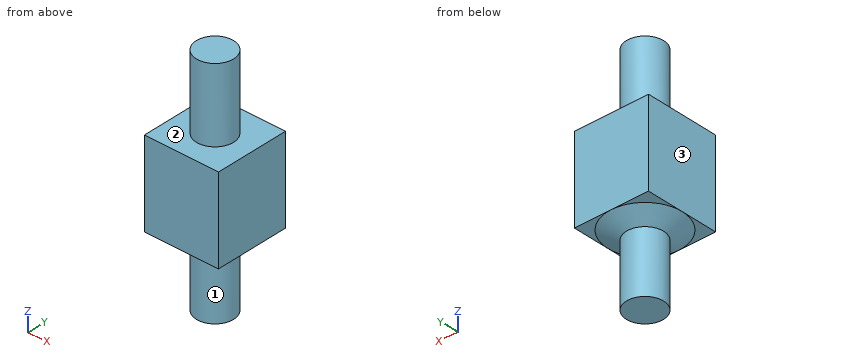
```python
from build123d import *

# Parameters (mm, degrees)
F0_R     = 2
F1_DEPTH = 25
F3_W     = 8
F3_H     = 8
F4_DEPTH = 9.3


with BuildPart() as f1:
    # F0 (on Top) → F1 (new body)
    with BuildSketch(Plane.XY):
        Circle(F0_R)
    extrude(amount=F1_DEPTH)

    # F3 (on offset) → F4 (join)
    with BuildSketch(Plane.XY.offset(17)):
        Rectangle(F3_W, F3_H)
    extrude(amount=-F4_DEPTH)

    # F5 (on Front) → F6 (revolve)
    with BuildSketch(Plane.XZ):
        Polygon((0, 7.7), (0, 5.7), (4, 7.7), align=None)
    revolve(axis=Axis((0, 0, 6.7), (0, 0, -1)))


solid = f1.part
```
Here's how the part is built. I have some questions about the finished solid (model axes, mm). Face numbers are marked on the shaded views. A direction names the side the tool comes from. Round coordinates to 2 decimals unless told otherwise and drop trailing zeros. Order: outer loops, then holes, each group sorted by start corner. A loop starts at its lowest first (then second) coordinate and runs counter-clockwise, first axis right, second up. Notation, with made-up numbers: M -39,-21 L 20,-21 A19 ccw 20,-3 Z; hole C -12,10.5 d8. An arc over 180 degrees is marked long. Answer in a Markdown table with one row per item.
Item 1: For the marked faces 1, 2 and 3, which set-ups out of +Z, -Z, +X, -X, +Y, -Y let a thin tool reach every point of the face, with its end or its side?
A:
| item | result |
|---|---|
| face 1 | -Z |
| face 2 | +Z |
| face 3 | +Z, -Z, -X, +Y, -Y |
Item 2: I'm going to push flat-ended pins straight in: pin 1 (2 mm diameter, centred on x = -2, y = -3, fed in from -Z); pin 2 (1.2 mm diameter, centred on x = -1.5, y = -2.5, fed in from -Z); pin 3 (1 mm diameter, centred on y = 0.5, z = 3.5, fed in from -X). Where does each tip first touch, or does it pass through?
A:
| item | result |
|---|---|
| pin 1 | stops at z = 7 |
| pin 2 | stops at z = 6.86 |
| pin 3 | stops at x = -2 |
Item 3: If I drill on L1, parallel to Z at x = -3, y = -3; L2, parallel to Y at x = 0, z = 19.5; L3, parallel to Z at x = -1, y = 2, over which ranges is the centre line in solid material (lowest first)? Write a range as from..to.
A:
| item | result |
|---|---|
| L1 | z = 7.7..17 |
| L2 | y = -2..2 |
| L3 | z = 6.82..17 |
Item 4: Imagine slicing it at A-A, the plane z = 20.5. Write out the boundary of the cut face in (x, y), and give its area (3 significant figures).
A:
| item | result |
|---|---|
| outline | C 0,0 d4 |
| area | 12.6 mm2 |
